Could you check a few things on this model? Use its own coordinates, in mm. Face numbers are marked on the shaded views. A direction names the side the tool comes from. Give positions to 0.01 mm unless a question says otherwise; leave off trailing zeros. Loops run counter-clockwise (first coordinate to the right, second up) from the corner with the lowest first, then second, coordinate; pieces in that order, holes last. Notation, with made-up numbers: M 84.25,61 L 119.25,61 A31 cw 119.25,86 Z; hole C -27,71.25 d7. An arc over 180 degrees is marked long. Return JSON: item names as keys, results as strings. Group by question number.
1. If we section it at B-B (y = -37): Write out the boundary of the cut face in (x, z), plus the area to 3 significant figures.
2. Please list where these lines run through material, in increasing order: line 1 (Y direction, x = -1.5, z = 9); line 2 (Y direction, x = 37.5, z = 8); line 3 (X direction, y = -34, z = 26.5).
3. If we section it at D-D (z = 21): Write out the boundary of the cut face in (x, y), plus the area to 3 significant figures.
4. If we mould it in two halves opening along Y, with no side actions, what happens to the marked faces 4, 5 and 6? For each: +Y half, -Y half, draft (parallel to the pull), parting line (faces both ways), or undercut.
5. For pin 1 (1.5 mm diameter, centred on x = 36, y = -54, fed in from +Z); pin 2 (5 mm diameter, centred on x = 16, y = -52, fed in from +Z); pin 3 (3.5 mm diameter, centred on x = 42.3, y = -45.29, fed in from -Z), each with a flat end and sliding along its axis, tell me the tip position at first contact or that it passes through.
6. If we section it at C-C (x = 31): Write out the boundary of the cut face in (y, z), plus the area to 3 significant figures.
7. For the marked faces 1, 2 and 3, which set-ups out of +Z, -Z, +X, -X, +Y, -Y let a thin tool reach every point of the face, with its end or its side?
8. If we section it at A-A (x = 13.5): Write out the boundary of the cut face in (y, z).
```python
from build123d import *

# Parameters (mm, degrees)
SKETCH3_W               = 5
SKETCH3_H               = 41
SKETCH3_W_2             = 40.6
SKETCH3_H_2             = 5.921911982
SKETCH3_H_3             = 5.716066276
BOSS_EXTRUDE3_DEPTH     = 29.5
SKETCH4_W               = 38
SKETCH4_H               = 19.5
CUT_EXTRUDE1_DEPTH      = 83
SKETCH6_W               = 2
SKETCH6_H               = 62.25
BOSS_EXTRUDE4_DEPTH     = 30
CUT_EXTRUDE3_DEPTH      = 96.683171243
CUT_EXTRUDE3_DEPTH_BACK = 77
SKETCH9_W               = 24.4
SKETCH9_H               = 17.5
SKETCH10_R              = 2
BOSS_EXTRUDE5_DEPTH     = 12
CUT_EXTRUDE4_DEPTH      = 29
SKETCH12_W              = 5
SKETCH12_H              = 3.036960159
CUT_EXTRUDE5_DEPTH      = 66
SKETCH13_R              = 1.575
CUT_EXTRUDE6_DEPTH      = 20
BOSS_EXTRUDE6_DEPTH     = 7
FILLET1_R               = 10
SKETCH15_R              = 2.1
CUT_EXTRUDE7_DEPTH      = 13
SKETCH16_W              = 37
SKETCH16_H              = 62.25
BOSS_EXTRUDE7_DEPTH     = 2
BOSS_EXTRUDE8_DEPTH     = 4
SKETCH19_W              = 40.6
SKETCH19_H              = 3.403788035
CUT_EXTRUDE8_DEPTH      = 97.335783039
SKETCH20_W              = 5.557340338
SKETCH20_H              = 21.5
BOSS_EXTRUDE9_DEPTH     = 66.25
SKETCH22_R              = 2
CUT_EXTRUDE11_DEPTH     = 12


with BuildPart() as part:
    # Sketch3 → Boss-Extrude3 (new body)
    with BuildSketch(Plane.XY):
        Polygon((37.007505292, -41.485394176), (37.007505292, -0.485394176), (37.007505292, 10.139605824), (32.007505292, 10.139605824), (32.007505292, 4.217693842), (32.007505292, -46.3943279), (32.007505292, -52.110394176), (37.007505292, -52.110394176), align=None)
        with Locations((63.907505292, -20.985394176)):
            Rectangle(SKETCH3_W, SKETCH3_H)
        Polygon((61.407505292, -41.485394176), (37.007505292, -41.485394176), (37.007505292, -52.110394176), (66.407505292, -52.110394176), (66.407505292, -41.485394176), align=None)
        Polygon((37.007505292, 10.139605824), (37.007505292, -0.485394176), (61.407505292, -0.485394176), (66.407505292, -0.485394176), (66.407505292, 10.139605824), align=None)
        with Locations((11.707505292, 7.178649833)):
            Rectangle(SKETCH3_W_2, SKETCH3_H_2)
        with Locations((11.707505292, -49.252361038)):
            Rectangle(SKETCH3_W_2, SKETCH3_H_3)
    extrude(amount=BOSS_EXTRUDE3_DEPTH)

    # Sketch4 → Cut-Extrude1 (cut)
    with BuildSketch(Plane.XZ.offset(52.110394176)):
        with Locations((10.407505292, 19.75)):
            Rectangle(SKETCH4_W, SKETCH4_H)
    extrude(amount=-CUT_EXTRUDE1_DEPTH, mode=Mode.SUBTRACT)

    # Sketch6 → Boss-Extrude4 (add)
    with BuildSketch(Plane(origin=(66.407505292, 0, 0), x_dir=(0, 0, -1), z_dir=(1, 0, 0))):
        with Locations((-28.5, -20.985394176)):
            Rectangle(SKETCH6_W, SKETCH6_H)
    extrude(amount=-BOSS_EXTRUDE4_DEPTH)

    # Sketch9 → Cut-Extrude3 (cut, two sides: drawn at the far end of the back side and taken through both)
    with BuildSketch(Plane(origin=(0, -52.110394176, 0), x_dir=(-1, 0, 0), z_dir=(0, -1, 0)).offset(-CUT_EXTRUDE3_DEPTH_BACK)):
        with Locations((-49.207505292, -18.75)):
            Rectangle(SKETCH9_W, SKETCH9_H)
    extrude(amount=CUT_EXTRUDE3_DEPTH + CUT_EXTRUDE3_DEPTH_BACK, mode=Mode.SUBTRACT)

    # Sketch10 → Boss-Extrude5 (add)
    with BuildSketch(Plane.XY.offset(29.5)):
        with Locations((51.407505292, -32.900394176)):
            Circle(SKETCH10_R)
    extrude(amount=BOSS_EXTRUDE5_DEPTH)

    # Sketch11 → Cut-Extrude4 (cut)
    with BuildSketch(Plane(origin=(66.407505292, 0, 0), x_dir=(0, 0, -1), z_dir=(1, 0, 0))):
        Polygon((0, -41.485394176), (-9.829517325, -41.485394176), (-9.829517325, -52.110394176), (-24.463039841, -52.110394176), (-24.463039841, -42.110394176), (-24.463039841, 0), (-24.463039841, 10.139605824), (-9.829517325, 10.139605824), (-9.829517325, 0.139605824), (0, 0.139605824), align=None)
    extrude(amount=-CUT_EXTRUDE4_DEPTH, mode=Mode.SUBTRACT)

    # Sketch12 → Cut-Extrude5 (cut)
    with BuildSketch(Plane(origin=(0, 10.139605824, 0), x_dir=(1, 0, 0), z_dir=(0, 1, 0))):
        with Locations((63.907505292, -25.98151992)):
            Rectangle(SKETCH12_W, SKETCH12_H)
    extrude(amount=-CUT_EXTRUDE5_DEPTH, mode=Mode.SUBTRACT)

    # Sketch13 → Cut-Extrude6 (cut)
    with BuildSketch(Plane(origin=(0, 10.139605824, 0), x_dir=(1, 0, 0), z_dir=(0, 1, 0))):
        with Locations(Location((-1.592494708, -4.992044142, 0), (0, 0, 180))):
            Circle(SKETCH13_R)
        with Locations(Location((8.567505292, -4.980496782, 0), (0, 0, 180))):
            Circle(SKETCH13_R)
    extrude(amount=-CUT_EXTRUDE6_DEPTH, mode=Mode.SUBTRACT)

    # Sketch14 → Boss-Extrude6 (add)
    with BuildSketch(Plane(origin=(0, 10.139605824, 0), x_dir=(1, 0, 0), z_dir=(0, 1, 0))):
        Polygon((47.007505292, -27.5), (37.007505292, -14.894614106), (37.007505292, -27.5), align=None)
    extrude(amount=-BOSS_EXTRUDE6_DEPTH)

    # Fillet1
    fillet1_edges = [part.edges().sort_by_distance(p)[0] for p in [
        (47.007505292, 6.639605824, 27.5),
        (37.007505292, 6.639605824, 14.894614106),
    ]]
    fillet(fillet1_edges, radius=FILLET1_R)

    # Sketch15 → Cut-Extrude7 (cut)
    with BuildSketch(Plane(origin=(0, 0, 0), x_dir=(-1, 0, 0), z_dir=(0, 0, -1))):
        with Locations((-42.297505292, -45.285394176)):
            Circle(SKETCH15_R)
        with Locations((-52.297505292, -45.285394176)):
            Circle(SKETCH15_R)
        with Locations((-42.297505292, 3.314605824)):
            Circle(SKETCH15_R)
        with Locations((-52.297505292, 3.314605824)):
            Circle(SKETCH15_R)
    extrude(amount=-CUT_EXTRUDE7_DEPTH, mode=Mode.SUBTRACT)

    # Sketch16 → Boss-Extrude7 (add)
    with BuildSketch(Plane.XY.offset(29.5)):
        with Locations((47.907505292, -20.985394176)):
            Rectangle(SKETCH16_W, SKETCH16_H)
    extrude(amount=BOSS_EXTRUDE7_DEPTH)

    # Sketch17 → Boss-Extrude8 (add)
    with BuildSketch(Plane.XZ.offset(52.110394176)):
        Polygon((-8.592494708, 0), (66.407505292, 0), (66.407505292, 9.829517325), (37.407505292, 9.829517325), (37.407505292, 10), (37.007505292, 10), (37.007505292, 27.5), (66.407505292, 27.5), (66.407505292, 31.5), (37.007505292, 31.5), (37.007505292, 31.503473539), (35.075655428, 31.503473539), (35.075655428, 10), (-8.592494708, 10), align=None)
    extrude(amount=BOSS_EXTRUDE8_DEPTH)

    # Sketch19 → Cut-Extrude8 (cut, through all)
    with BuildSketch(Plane(origin=(0, 0, 0), x_dir=(-1, 0, 0), z_dir=(0, 0, -1))):
        with Locations((-11.707505292, -48.096221918)):
            Rectangle(SKETCH19_W, SKETCH19_H)
    extrude(amount=-CUT_EXTRUDE8_DEPTH, mode=Mode.SUBTRACT)

    # Sketch20 → Boss-Extrude9 (add)
    with BuildSketch(Plane(origin=(0, 10.139605824, 0), x_dir=(1, 0, 0), z_dir=(0, 1, 0))):
        with Locations((32.186175461, -20.75)):
            Rectangle(SKETCH20_W, SKETCH20_H)
    extrude(amount=-BOSS_EXTRUDE9_DEPTH)

    # Sketch22 → Cut-Extrude11 (cut)
    with BuildSketch(Plane.XZ.offset(56.110394176)):
        with Locations(Location((-1.992494708, 4.992044142, 0), (0, 0, 270))):
            Circle(SKETCH22_R)
    extrude(amount=-CUT_EXTRUDE11_DEPTH, mode=Mode.SUBTRACT)


solid = part.part
```
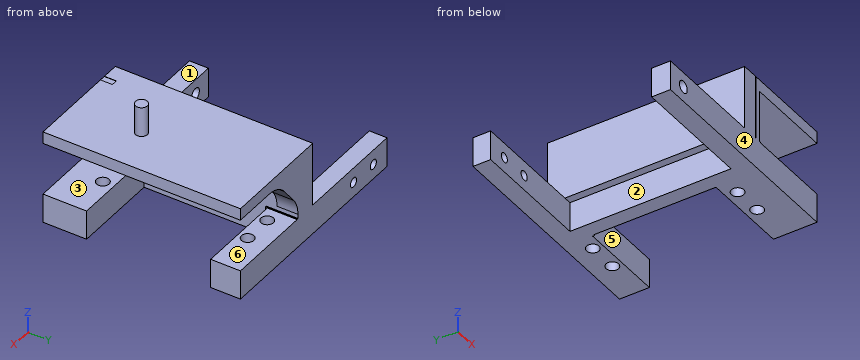
Answer:
{
 "1": {"outline": "M 29.41,10 L 32.01,10 L 32.01,0 L 37.01,0 L 37.01,27.5 L 66.41,27.5 L 66.41,31.5 L 29.41,31.5 Z", "area": "331 mm²"},
 "2": {"line 1": "y = -56.11 to -49.8, 4.22 to 10.14", "line 2": "y = -56.11 to -41.49, 0.14 to 10.14", "line 3": "x = 29.41 to 37.01"},
 "3": {"outline": "M 29.41,-56.11 L 34.96,-56.11 L 34.96,-52.11 L 35.08,-52.11 L 35.08,-56.11 L 37.01,-56.11 L 37.01,3.14 L 41.85,3.14 L 41.85,10.14 L 29.41,10.14 Z", "area": "537 mm²"},
 "4": {"face 4": "-Y half", "face 5": "undercut", "face 6": "draft"},
 "5": {"pin 1": "stops at z = 31.5", "pin 2": "stops at z = 10", "pin 3": "stops at z = 27.5"},
 "6": {"outline": "M -56.11,0 L -49.8,0 L -49.8,10 L 4.22,10 L 4.22,0 L 10.14,0 L 10.14,31.5 L -56.11,31.5 Z", "area": "1,550 mm²"},
 "7": {"face 1": "+Z, -X, +Y, -Y", "face 2": "-Z, -X", "face 3": "+X, +Y, -Y"},
 "8": {"outline": "M -56.11,0 L -49.8,0 L -49.8,10 L -56.11,10 Z; M 4.22,0 L 10.14,0 L 10.14,10 L 4.22,10 Z"}
}
